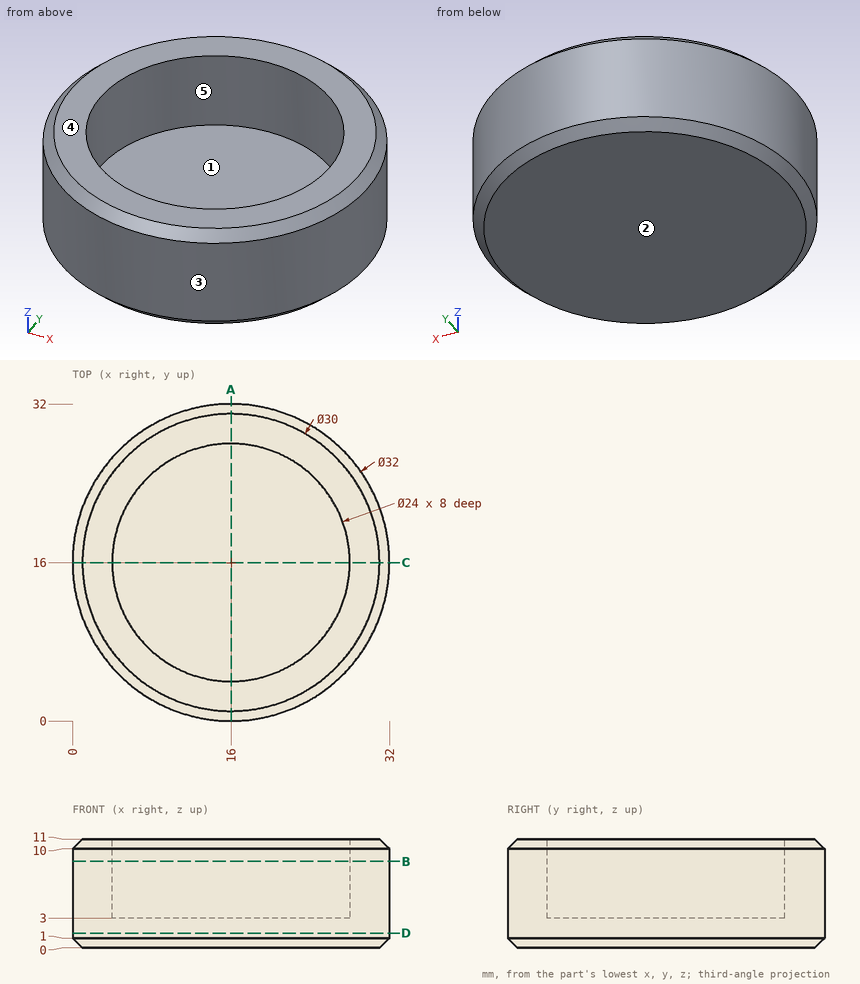
Geometry check sheet. Reference: drawing and pictorial views, mm from the part's lowest x, y, z. A direction names the side the tool comes from. Round coordinates to 2 decimals unless told otherwise and drop trailing zeros. Loops run counter-clockwise (first coordinate to the right, second up) from the corner with the lowest first, then second, coordinate; pieces in that order, holes last. Notation, with made-up numbers: (8, -28.75) - (46, -28.75) arc R19 cw to (46, 0.25) - close; hole circle Ø6 at (-10, 69.25). An arc over 180 degrees is marked (long way). Answer in a Markdown table with one row per item. Add a question column.
Q1. Tool access check on the marked faces 4 and 5. Record the directions out of +Z, -Z, +X, -X, +Y, -Y that give a thin tool (end or side, any length) a straight path to the whole face; none if there is none.
Q2. Material ranges on line 1 (Y direction, x = 16, z = 7); line 2 (Z direction, x = 12.5, y = 18.5); line 3 (X direction, y = 8, z = 4), recorded low to high.
Q3. Section check D-D on z = 1.5. Enter the section's corners in (x, y).
Q4. Gauge pin test, flat ends, axial feed: pin 1 (3 mm diameter, centred on y = 24, z = 9, fed in from +X); pin 2 (4 mm diameter, centred on x = 26, z = 9.5, fed in from +Y); pin 3 (6 mm diameter, centred on x = 8, y = 12.5, fed in from -Z); pin 4 (4 mm diameter, centred on x = 21.5, z = 9, fed in from +Y). Record the tip position at first contact, or that the pin passes through.
Q5. Section check B-B on z = 8.75. Enter the section's corners in (x, y).
Q6. Section check A-A on x = 16. Enter the section's corners in (y, z), plus the area to 3 significant figures.
Q7. Release check for a two-part mould opening along X. For the marked faces 1, 2 and 3 record: pulls with the +X half, pulls with the -X half, needs draft (parallel to the pull), parting line crosses it, or undercut.
Found:
| question | item | result |
|---|---|---|
| 1 | face 4 | +Z, +X, -X, +Y, -Y |
| 1 | face 5 | +Z |
| 2 | line 1 | y = 0 to 4, 28 to 32 |
| 2 | line 2 | z = 0 to 3 |
| 2 | line 3 | x = 2.14 to 7.06, 24.94 to 29.86 |
| 3 | outline | circle Ø32 at (16, 16) |
| 4 | pin 1 | stops at x = 30.62 |
| 4 | pin 2 | stops at y = 29.86 |
| 4 | pin 3 | stops at z = 0 |
| 4 | pin 4 | stops at y = 31.61 |
| 5 | outline | circle Ø32 at (16, 16); hole circle Ø24 at (16, 16) |
| 6 | outline | (0, 1) - (1, 0) - (31, 0) - (32, 1) - (32, 10) - (31, 11) - (28, 11) - (28, 3) - (4, 3) - (4, 11) - (1, 11) - (0, 10) - close |
| 6 | area | 158 mm² |
| 7 | face 1 | undercut |
| 7 | face 2 | needs draft |
| 7 | face 3 | parting line crosses it |
